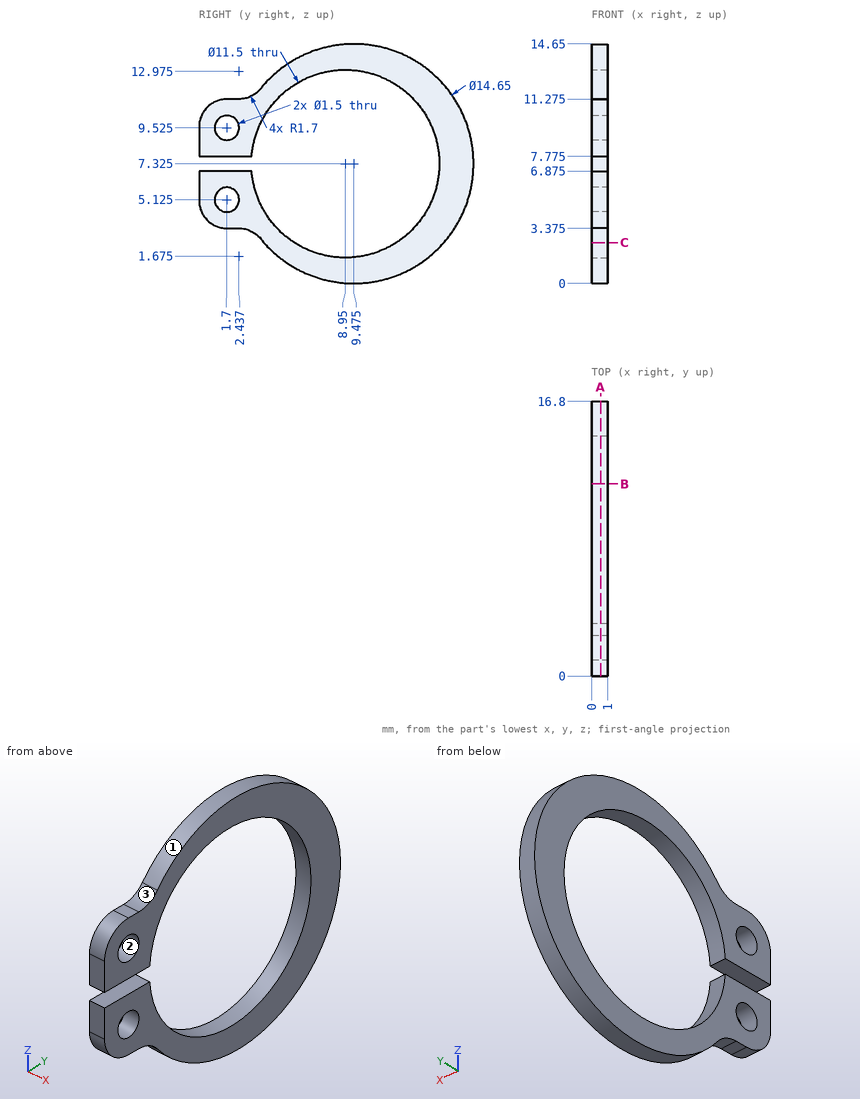
Drawing for the job (mm, zero at the part's lowest x, y, z). Round coordinates to 2 decimals unless told otherwise and drop trailing zeros. Order: outer loops, then holes, each group sorted by start corner. A loop starts at its lowest first (then second) coordinate and runs counter-clockwise, first axis right, second up.
Item 1: Mould opens along Z. For the marked faces 1, 2 and 3 say: pulls with the +Z half, pulls with the -Z half, needs draft (parallel to the pull), parting line crosses it, or undercut.
Item 2: Saw through at C-C on z = 2.5. Write the cut outline in (x, y).
Item 3: Saw through at A-A on x = 0.55. State how many separate pieces and enclosed holes the cut face has.
Item 4: Saw through at B-B on y = 11.75. Write the cut outline in (x, z).
Item 5: Pin check, flat tips, straight feed: pin 1 (1.7 mm diameter, centred on y = 1.7, z = 5.125, fed in from +X); pin 2 (0.6 mm diameter, centred on x = 0.5, y = 2, fed in from -Z) (3 decimals). Stop position of each tip, or through.
Item 6: Probe line 1 along Z through (x, y) = (0.65, 2.75) (1 decimal); line 2 along Z through (x, y) = (0.2, 3.75) (1 decimal); line 3 along Y through (x, z) = (0.2, 3) (1 decimal). List the from-to ranges inside material, lowest first.
Reported:
1. face 1: parting line crosses it
1. face 2: undercut
1. face 3: pulls with the +Z half
2. outline: (0, 3.96) - (1, 3.96) - (1, 5.82) - (0, 5.82) - close; (0, 12.08) - (1, 12.08) - (1, 14.99) - (0, 14.99) - close
3. separate pieces: 1
3. enclosed holes: 2
4. outline: (0, 0.36) - (1, 0.36) - (1, 2.3) - (0, 2.3) - close; (0, 12.35) - (1, 12.35) - (1, 14.29) - (0, 14.29) - close
5. pin 1: stops at x = 1
5. pin 2: stops at z = 3.375
6. line 1: z = 3.3 to 6.9, 7.8 to 11.3
6. line 2: z = 2.8 to 4.9, 9.8 to 11.9
6. line 3: y = 3.5 to 5.2, 12.7 to 15.4
